Input: part model. Units: mm. Frame: model coordinates. Coordinates: 2 decimals unless noted, no trailing zeros. Loops run counter-clockwise (first coordinate to the right, second up) from the corner with the lowest first, then second, coordinate; pieces in that order, holes last.
```python
from build123d import *

# Parameters (mm, degrees)
BASISTEIL_BECHER_1_START       = -43
BASISTEIL_BECHER_1_OUTLINE_R   = 32.5
BASISTEIL_BECHER_1_OUTLINE_R_2 = 1.75
BASISTEIL_BECHER_1_OUTLINE_R_3 = 27.5
BASISTEIL_BECHER_1_DEPTH       = 3
CUT_EXTRUDE1_START             = -0.5
SKETCH1_R                      = 32.5
CUT_EXTRUDE1_DEPTH             = 0.5
BOSS_EXTRUDE1_START            = -2.5
SKETCH3_R                      = 33
SKETCH3_R_2                    = 32.5
BOSS_EXTRUDE1_DEPTH            = 2.5
CHAMFER1_SIZE                  = 0.6


# Read off the part's stored shape, not the designer's step: Basisteil-Becher-1
with BuildPart() as part:
    # Basisteil-Becher-1 outline → Basisteil-Becher-1 (new body)
    with BuildSketch(Plane(origin=(0, 0, 0), x_dir=(1, 0, 0), z_dir=(0, 1, 0)).offset(BASISTEIL_BECHER_1_START)):
        Circle(BASISTEIL_BECHER_1_OUTLINE_R)
        with Locations((-15, -25.980762114)):
            Circle(BASISTEIL_BECHER_1_OUTLINE_R_2, mode=Mode.SUBTRACT)
        with Locations((-25.980762114, -15)):
            Circle(BASISTEIL_BECHER_1_OUTLINE_R_2, mode=Mode.SUBTRACT)
        with Locations((0, -30)):
            Circle(BASISTEIL_BECHER_1_OUTLINE_R_2, mode=Mode.SUBTRACT)
        with Locations((15, -25.980762114)):
            Circle(BASISTEIL_BECHER_1_OUTLINE_R_2, mode=Mode.SUBTRACT)
        with Locations((25.980762114, -15)):
            Circle(BASISTEIL_BECHER_1_OUTLINE_R_2, mode=Mode.SUBTRACT)
        with Locations((-30, 0)):
            Circle(BASISTEIL_BECHER_1_OUTLINE_R_2, mode=Mode.SUBTRACT)
        with Locations((-25.980762114, 15)):
            Circle(BASISTEIL_BECHER_1_OUTLINE_R_2, mode=Mode.SUBTRACT)
        with Locations((-15, 25.980762114)):
            Circle(BASISTEIL_BECHER_1_OUTLINE_R_2, mode=Mode.SUBTRACT)
        Circle(BASISTEIL_BECHER_1_OUTLINE_R_3, mode=Mode.SUBTRACT)
        with Locations((30, 0)):
            Circle(BASISTEIL_BECHER_1_OUTLINE_R_2, mode=Mode.SUBTRACT)
        with Locations((25.980762114, 15)):
            Circle(BASISTEIL_BECHER_1_OUTLINE_R_2, mode=Mode.SUBTRACT)
        with Locations((0, 30)):
            Circle(BASISTEIL_BECHER_1_OUTLINE_R_2, mode=Mode.SUBTRACT)
        with Locations((15, 25.980762114)):
            Circle(BASISTEIL_BECHER_1_OUTLINE_R_2, mode=Mode.SUBTRACT)
    extrude(amount=BASISTEIL_BECHER_1_DEPTH)

    # Sketch1 → Cut-Extrude1 (cut)
    with BuildSketch(Plane(origin=(0, -40, 0), x_dir=(1, 0, 0), z_dir=(0, 1, 0)).offset(CUT_EXTRUDE1_START)):
        with Locations(Location((0, 0, 0), (0, 0, 270))):
            Circle(SKETCH1_R)
    extrude(amount=CUT_EXTRUDE1_DEPTH, mode=Mode.SUBTRACT)

    # Sketch3 → Boss-Extrude1 (add)
    with BuildSketch(Plane(origin=(0, -40.5, 0), x_dir=(1, 0, 0), z_dir=(0, 1, 0)).offset(BOSS_EXTRUDE1_START)):
        with Locations(Location((0, 0, 0), (0, 0, 270))):
            Circle(SKETCH3_R)
        Circle(SKETCH3_R_2, mode=Mode.SUBTRACT)
    extrude(amount=BOSS_EXTRUDE1_DEPTH)

    # Chamfer1
    chamfer1_edges = [part.edges().sort_by_distance(p)[0] for p in [
        (0, -43, -33),
    ]]
    chamfer(chamfer1_edges, length=CHAMFER1_SIZE)


solid = part.part
```
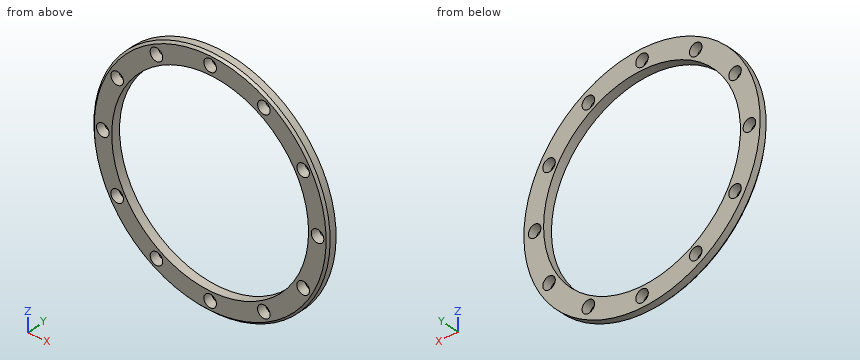
Item 1: Section query B-B (x = 0). Output: boundary loops of the cut face in (y, z), then the cut area to 3 significant figures.
Result:
outline: (-43, -32.4) - (-42.4, -33) - (-40.5, -33) - (-40.5, -31.75) - (-43, -31.75) - close; (-43, -28.25) - (-40.5, -28.25) - (-40.5, -27.5) - (-43, -27.5) - close; (-43, 27.5) - (-40.5, 27.5) - (-40.5, 28.25) - (-43, 28.25) - close; (-43, 31.75) - (-40.5, 31.75) - (-40.5, 33) - (-42.4, 33) - (-43, 32.4) - close
area: 9.64 mm2
Item 2: Contact query for flat-ended pins moving along their axis: P1, Ø3, axis at x = 15, z = -25.98, coming from the -Y side; P2, Ø1, axis at x = -12.5, y = -42, coming from the +Z side. Output: stop coordinate, or through.
Result:
P1: passes through
P2: stops at z = 30.74
Item 3: Line query: L1, parallel to X at y = -42, z = 13.5; L2, parallel to Z at x = 15, y = -42.4; L3, parallel to X at y = -40.65, z = 16. Output: solid intervals per line, ascending.
Result:
L1: x = -30.11 to -26.88, -25.08 to -23.96, 23.96 to 25.08, 26.88 to 30.11
L2: z = -29.39 to -27.73, -24.23 to -23.05, 23.05 to 24.23, 27.73 to 29.39
L3: x = -28.86 to -27.42, -24.54 to -22.37, 22.37 to 24.54, 27.42 to 28.86
Item 4: Section query A-A (z = 0). Output: boundary loops of the cut face in (x, y).
Result:
outline: (-33, -42.4) - (-32.4, -43) - (-31.75, -43) - (-31.75, -40.5) - (-33, -40.5) - close; (-28.25, -43) - (-27.5, -43) - (-27.5, -40.5) - (-28.25, -40.5) - close; (27.5, -43) - (28.25, -43) - (28.25, -40.5) - (27.5, -40.5) - close; (31.75, -43) - (32.4, -43) - (33, -42.4) - (33, -40.5) - (31.75, -40.5) - close
Item 5: Section query C-C (y = -41.9). Count the separate pieces of the cut face and the enclosed holes in it, then the cut area to 3 significant figures.
Result:
separate pieces: 1
enclosed holes: 13
area: 930 mm2
